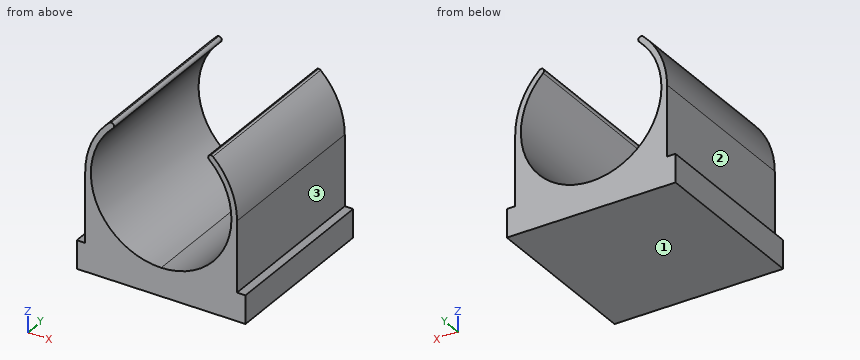
```python
from build123d import *

# Parameters (mm, degrees)
F1_W     = 30
F1_H     = 30
F2_DEPTH = 5
F3_DEPTH = 15
F4_R     = 0.49999


# Not quite as in the source:
# - a fillet or chamfer is up to 0.001 mm smaller than in the source, because OpenCascade refuses the exact size


with BuildPart() as f2:
    # F1 (on Top) → F2 (new body)
    with BuildSketch(Plane.XY):
        Rectangle(F1_W, F1_H)
    extrude(amount=-F2_DEPTH)

    # F0 (on Front) → F3 (join, symmetric)
    with BuildSketch(Plane.XZ):
        with BuildLine():
            ThreePointArc((0, 0), (-11.8585412256, 8.5471529248), (-7.5, 22.5))
            Line((-7.5, 22.5), (-9.0691785736, 22.5))
            ThreePointArc((-9.0691785736, 22.5), (-12.3426883365, 17.9688247941), (-13.5, 12.5))
            Line((-13.5, 12.5), (-13.5, 0))
            Line((-13.5, 0), (0, 0))
        make_face()
        with BuildLine():
            ThreePointArc((7.5, 22.5), (11.8585412256, 8.5471529248), (0, 0))
            Line((0, 0), (13.5, 0))
            Line((13.5, 0), (13.5, 12.5))
            ThreePointArc((13.5, 12.5), (12.3426883365, 17.9688247941), (9.0691785736, 22.5))
            Line((9.0691785736, 22.5), (7.5, 22.5))
        make_face()
    extrude(amount=F3_DEPTH, both=True)

    # F4 (radius 0.5 in the source; OpenCascade refuses exactly that, so slightly less here)
    f4_edges = [f2.edges().sort_by_distance(p)[0] for p in [
        (-7.5, 0, 22.5),
        (9.069179, 0, 22.5),
        (-9.069179, 0, 22.5),
        (7.5, 0, 22.5),
    ]]
    fillet(f4_edges, radius=F4_R)


solid = f2.part
```
The listing builds one solid part. Answer for the finished solid, in the listing's coordinates (mm). Face numbers are marked on the shaded views. A direction names the side the tool comes from. Round coordinates to 2 decimals unless told otherwise and drop trailing zeros. Write each loop counter-clockwise with the first axis right and the second up, starting at its lowest first coordinate (ties: lowest second). Pieces come first, ordered by that corner, then holes. Notation, with made-up numbers: (19, -16) -> (50, -16) arc R19 ccw to (50, -11) -> close; hole circle Ø7 at (25.5, -16.5). An arc over 180 degrees is marked (long way). Use CSV: the item, a comma, the result in double quotes. Start each with the question number.
(1) Section A-A on z = 0.5 is taken. Give the vertices of the cut face in (x, y), then the cut area to 3 significant figures.
(2) Section D-D on x = -6.5 is taken. Give the vertices of the cut face in (y, z).
(3) Consider L1, parallel to X at y = 5.5, z = 12.75; L2, parallel to X at y = 10.75, z = 15.5; L3, parallel to Z at x = 10.75, y = -9.25. Determine where each line is inside the solid, lowest interval first. Write a range as from..to.
(4) Which of the six approach directions +Z, -Z, +X, -X, +Y, -Y give full straight-line access (tool end or side, diameter ignored) to the marked faces 1, 2 and 3?
(5) Each of these flat-tipped pins is pushed along its axis until it touches: pin 1 (4 mm diameter, centred on y = 5, z = 8, fed in from -X); pin 2 (2 mm diameter, centred on x = 10, y = -6.5, fed in from +Z); pin 3 (4 mm diameter, centred on y = -3, z = 8.5, fed in from +X). Where does it stop, or does it pass through?
(6) Section B-B on x = 11.75 is taken. Give the vertices of the cut face in (y, z).
A:
1,outline,"(-13.5, -15) -> (-3.5, -15) -> (-3.5, 15) -> (-13.5, 15) -> close; (3.5, -15) -> (13.5, -15) -> (13.5, 15) -> (3.5, 15) -> close"
1,area,"600 mm²"
2,outline,"(-15, -5) -> (15, -5) -> (15, 1.82) -> (-15, 1.82) -> close"
3,L1,"x = -13.5..-12.5, 12.5..13.5"
3,L2,"x = -13.16..-12.13, 12.13..13.16"
3,L3,"z = -5..6.12, 18.88..20.67"
4,face 1,"-Z, +X, -X, +Y, -Y"
4,face 2,"+Z, -X, +Y, -Y"
4,face 3,"+Z, +X, +Y, -Y"
5,pin 1,"stops at x = -13.5"
5,pin 2,"stops at z = 22.48"
5,pin 3,"stops at x = 13.5"
6,outline,"(-15, -5) -> (15, -5) -> (15, 8.24) -> (-15, 8.24) -> close; (-15, 16.76) -> (15, 16.76) -> (15, 19.15) -> (-15, 19.15) -> close"
